Design review of the part built by this model. Coordinates are the model's own, in mm. A direction names the side the tool comes from. Round coordinates to 2 decimals unless told otherwise and drop trailing zeros. Write each loop counter-clockwise with the first axis right and the second up, starting at its lowest first coordinate (ties: lowest second). Pieces come first, ordered by that corner, then holes. Notation, with made-up numbers: M 28.25,-5.75 L 81.25,-5.75 A13 cw 81.25,-1.75 Z; hole C -6.5,7 d6. An arc over 180 degrees is marked long. One line per question, with ' | ' between items. Start each with the question number.
Item 1: For L1, parallel to Y at x = 42, z = 2.35; L2, parallel to Y at x = 41.25, z = 0.75; L3, parallel to X at y = 115, z = 1.55, list the stretches that pass through material, from the lowest coordinate up.
Item 2: Draft analysis for pull direction X (two halves, no side actions). For faces 3 (the face through (-1, 5, 0)), 4 (the face through (-37.591, 123.862, 1.479)), state which applies: released by +X, released by -X, zero draft, split by the parting line, or undercut.
Item 3: Add section A-A, the plane x = -6. State the section outline as (y, z) points, and give its area (3 significant figures).
Item 4: Machinability: for faces 1 (the face through (37.591, 49.138, 1.479)), 2 (the face through (-1, 5, 3)), which of the approach directions +Z, -Z, +X, -X, +Y, -Y give a long, thin tool a straight path to every point of the face, cutting with its end or side? Answer none if there is none.
Item 5: Add section B-B, the plane z = 1.05. Give the number of separate pieces and of enclosed holes in the cut face, and give its area (3 significant figures).
Autodesk Inventor part; units mm, degrees
ref_plane "YZ Plane" through (0, 0, 0) normal (1, 0, 0) x (0, 1, 0)
ref_plane "XZ Plane" through (0, 0, 0) normal (0, 1, 0) x (-1, 0, 0)
ref_plane "XY Plane" through (0, 0, 0) normal (0, 0, 1) x (1, 0, 0)
sketch "スケッチ1" plane through (0, 0, 0) normal (0, 0, 1) x (1, 0, 0)
  line L0 (-55, -225) -> (55, -225)
  line L1 (55, -225) -> (55, 225)
  line L2 (55, 225) -> (-55, 225)
  line L3 (-55, 225) -> (-55, -225)
  line L4 (-55, -225) -> (55, 225) construction
  line L5 (55, -225) -> (-55, 225) construction
  line L6 (-55, 195) -> (-50, 195) construction
  line L7 (-50, 195) -> (-25, 220) construction
  line L8 (-25, 220) -> (-25, 225) construction
  line L9 (-46, 40.5) -> (46, 40.5) construction
  line L10 (46, 40.5) -> (46, 132.5) construction
  line L11 (46, 132.5) -> (-46, 132.5) construction
  line L12 (-46, 132.5) -> (-46, 40.5) construction
  line L13 (-46, 40.5) -> (46, 132.5) construction
  line L14 (46, 40.5) -> (-46, 132.5) construction
  line L15 (-46, 1.5) -> (46, 1.5) construction
  line L16 (46, 1.5) -> (46, 37.5) construction
  line L17 (46, 37.5) -> (-46, 37.5) construction
  line L18 (-46, 37.5) -> (-46, 1.5) construction
  line L19 (-46, 1.5) -> (46, 37.5) construction
  line L20 (46, 1.5) -> (-46, 37.5) construction
  line L21 (0, 0) -> (0, 86.5) construction
  circle A0 centre (0, 86.5) radius 53 construction
  line L22 (-44.7, 41.8) -> (44.7, 41.8) construction
  line L23 (44.7, 41.8) -> (44.7, 131.2) construction
  line L24 (44.7, 131.2) -> (-44.7, 131.2) construction
  line L25 (-44.7, 131.2) -> (-44.7, 41.8) construction
  line L26 (-44.7, 41.8) -> (44.7, 131.2) construction
  line L27 (44.7, 41.8) -> (-44.7, 131.2) construction
  arc A1 (-28.4765, 131.2) -> (-44.7, 114.9765) centre (0, 86.5) ccw
  arc A2 (-44.7, 58.0235) -> (-28.4765, 41.8) centre (0, 86.5) ccw
  arc A3 (28.4765, 41.8) -> (44.7, 58.0235) centre (0, 86.5) ccw
  arc A4 (44.7, 114.9765) -> (28.4765, 131.2) centre (0, 86.5) ccw
  line L28 (-28.4765, 131.2) -> (28.4765, 131.2)
  line L29 (-44.7, 114.9765) -> (-44.7, 58.0235)
  line L30 (-28.4765, 41.8) -> (28.4765, 41.8)
  line L31 (44.7, 58.0235) -> (44.7, 114.9765)
  line L32 (-41.25, 45.25) -> (41.25, 45.25) construction
  line L33 (41.25, 45.25) -> (41.25, 127.75) construction
  line L34 (41.25, 127.75) -> (-41.25, 127.75) construction
  line L35 (-41.25, 127.75) -> (-41.25, 45.25) construction
  line L36 (-41.25, 45.25) -> (41.25, 127.75) construction
  line L37 (41.25, 45.25) -> (-41.25, 127.75) construction
  circle A5 centre (-41.25, 127.75) radius 2.25
  circle A6 centre (-41.25, 45.25) radius 2.25
  circle A7 centre (41.25, 45.25) radius 2.25
  circle A8 centre (41.25, 127.75) radius 2.25
  circle A9 centre (-45, 215) radius 2.25
  circle A10 centre (45, 215) radius 2.25
  circle A11 centre (45, -215) radius 2.25
  circle A12 centre (-45, -215) radius 2.25
  circle A13 centre (-45, 0) radius 2.25 construction
  circle A14 centre (45, 0) radius 2.25 construction
  line L38 (-55, 0) -> (55, 0) construction
  circle A15 centre (-41.25, -49.75) radius 2.25
  arc A16 (-44.7, -36.9765) -> (-28.4765, -53.2) centre (0, -8.5) ccw
  line L39 (-28.4765, -53.2) -> (28.4765, -53.2)
  arc A17 (28.4765, -53.2) -> (44.7, -36.9765) centre (0, -8.5) ccw
  circle A18 centre (41.25, -49.75) radius 2.25
  line L40 (44.7, -36.9765) -> (44.7, 19.9765)
  circle A19 centre (41.25, 32.75) radius 2.25
  arc A20 (44.7, 19.9765) -> (28.4765, 36.2) centre (0, -8.5) ccw
  line L41 (-28.4765, 36.2) -> (28.4765, 36.2)
  circle A21 centre (-41.25, 32.75) radius 2.25
  arc A22 (-28.4765, 36.2) -> (-44.7, 19.9765) centre (0, -8.5) ccw
  line L42 (-44.7, 19.9765) -> (-44.7, -36.9765)
  circle A23 centre (-41.25, -144.75) radius 2.25
  arc A24 (-44.7, -131.9765) -> (-28.4765, -148.2) centre (0, -103.5) ccw
  line L43 (-28.4765, -148.2) -> (28.4765, -148.2)
  arc A25 (28.4765, -148.2) -> (44.7, -131.9765) centre (0, -103.5) ccw
  circle A26 centre (41.25, -144.75) radius 2.25
  line L44 (44.7, -131.9765) -> (44.7, -75.0235)
  circle A27 centre (41.25, -62.25) radius 2.25
  arc A28 (44.7, -75.0235) -> (28.4765, -58.8) centre (0, -103.5) ccw
  line L45 (-28.4765, -58.8) -> (28.4765, -58.8)
  circle A29 centre (-41.25, -62.25) radius 2.25
  arc A30 (-28.4765, -58.8) -> (-44.7, -75.0235) centre (0, -103.5) ccw
  line L46 (-44.7, -75.0235) -> (-44.7, -131.9765)
  point P0 (0, 19.5)
  point P1 (0, 19.5)
  dimension "d12" = 106
  dimension "d0" = 110
  dimension "d1" = 450
  dimension "d2" = 135
  dimension "d3" = 30
  dimension "d4" = 30
  dimension "d5" = 5
  dimension "d6" = 92
  dimension "d7" = 92
  dimension "d8" = 92
  dimension "d9" = 36
  dimension "d10" = 3
  dimension "d11" = 1.5
  dimension "d13" = 89.4
  dimension "d14" = 89.4
  dimension "d15" = 82.5
  dimension "d16" = 82.5
  dimension "d17" = 4.5
  dimension "d25" = 4.5
  dimension "d26" = 10
  dimension "d27" = 10
  dimension "d28" = 10
  dimension "d29" = 10
  dimension "d30" = 10
  dimension "d31" = 10
  dimension "d32" = 10
  dimension "d33" = 10
  dimension "d34" = 10
  dimension "d35" = 10
  dimension "d45" = 95
extrude "押し出し1" add sketch "スケッチ1" along normal blind 3 contours L3 L2 L1 L0 | A15 | L42 A22 L41 A20 L40 A17 L39 A16 | A18 | A19 | A21 | A23 | L46 A30 L45 A28 L44 A25 L43 A24 | A26 | A27 | A29
sketch "スケッチ2" plane through (0, 0, 3) normal (0, 0, 1) x (1, 0, 0)
  circle A0 centre (-45, 215) radius 2.25 construction
  circle A1 centre (45, -215) radius 2.25 construction
  circle A2 centre (-45, -215) radius 2.25 construction
  circle A3 centre (-43, 213) radius 2.75 construction
  line L0 (55, 225) -> (-55, 225)
  line L1 (-55, 225) -> (-55, -225)
  line L2 (-43.7153, 216.8472) -> (-41.4298, 215.2577)
  line L3 (-45.2577, 211.4298) -> (-46.8472, 213.7153)
  circle A4 centre (-45, 215) radius 2.25 construction
  arc A5 (-43.7153, 216.8472) -> (-46.8472, 213.7153) centre (-45, 215) ccw
  arc A6 (-45.2577, 211.4298) -> (-41.4298, 215.2577) centre (-43, 213) ccw
  line L4 (55, 225) -> (-55, 225) construction
  line L5 (0, 225) -> (0, -225) construction
  line L6 (-55, -225) -> (55, -225) construction
  line L7 (-55, 0) -> (55, 0) construction
  line L8 (55, -225) -> (55, 225) construction
  circle A7 centre (45, 215) radius 2.25 construction
  circle A8 centre (43, 213) radius 2.75 construction
  line L9 (43.7153, 216.8472) -> (41.4298, 215.2577)
  line L10 (45.2577, 211.4298) -> (46.8472, 213.7153)
  circle A9 centre (45, 215) radius 2.25 construction
  arc A10 (46.8472, 213.7153) -> (43.7153, 216.8472) centre (45, 215) ccw
  arc A11 (41.4298, 215.2577) -> (45.2577, 211.4298) centre (43, 213) ccw
  circle A12 centre (-45, -215) radius 2.25 construction
  circle A13 centre (-43, -213) radius 2.75 construction
  line L11 (-43.7153, -216.8472) -> (-41.4298, -215.2577)
  line L12 (-45.2577, -211.4298) -> (-46.8472, -213.7153)
  circle A14 centre (-45, -215) radius 2.25 construction
  arc A15 (-46.8472, -213.7153) -> (-43.7153, -216.8472) centre (-45, -215) ccw
  arc A16 (-41.4298, -215.2577) -> (-45.2577, -211.4298) centre (-43, -213) ccw
  circle A17 centre (45, -215) radius 2.25 construction
  line L13 (45.2577, -211.4298) -> (46.8472, -213.7153)
  arc A18 (45.2577, -211.4298) -> (41.4298, -215.2577) centre (43, -213) ccw
  circle A19 centre (43, -213) radius 2.75 construction
  line L14 (43.7153, -216.8472) -> (41.4298, -215.2577)
  circle A20 centre (45, -215) radius 2.25 construction
  arc A21 (43.7153, -216.8472) -> (46.8472, -213.7153) centre (45, -215) ccw
  point P0 (0, 0)
  dimension "d38" = 5.5
  dimension "d39" = 12
  dimension "d40" = 12
extrude "押し出し2" cut sketch "スケッチ2" against normal through all
sketch "スケッチ3" plane through (0, 0, 3) normal (0, 0, 1) x (1, 0, 0)
  line L0 (-55, -225) -> (55, -225) construction
  line L1 (-55, -221.5) -> (55, -221.5)
  line L2 (55, -221.5) -> (55, -225)
  line L3 (55, -225) -> (-55, -225)
  line L4 (-55, -225) -> (-55, -221.5)
  line L5 (-55, -221.5) -> (55, -225) construction
  line L6 (55, -221.5) -> (-55, -225) construction
  line L7 (0, -223.25) -> (0, -225) construction
  point P0 (0, 0)
  dimension "d50" = 3.5
  dimension "d51" = 110
extrude "押し出し3" cut sketch "スケッチ3" against normal through all
sketch "スケッチ4" plane through (0, 0, 3) normal (0, 0, 1) x (1, 0, 0)
  line L0 (-55, -221.5) -> (55, -221.5) construction
  line L1 (55, -221.5) -> (55, 225) construction
  line L2 (55, 225) -> (-55, 225) construction
  line L3 (-55, 225) -> (-55, -221.5) construction
  circle A0 centre (-41.25, 127.75) radius 2.25 construction
  circle A1 centre (-41.25, 45.25) radius 2.25 construction
  circle A2 centre (41.25, 45.25) radius 2.25 construction
  circle A3 centre (41.25, 127.75) radius 2.25 construction
  line L4 (43.7153, -216.8472) -> (41.4298, -215.2577) construction
  arc A4 (45.2577, -211.4298) -> (41.4298, -215.2577) centre (43, -213) ccw construction
  line L5 (45.2577, -211.4298) -> (46.8472, -213.7153) construction
  arc A5 (43.7153, -216.8472) -> (46.8472, -213.7153) centre (45, -215) ccw construction
  line L6 (-28.4765, 131.2) -> (28.4765, 131.2) construction
  arc A6 (44.7, 114.9765) -> (28.4765, 131.2) centre (0, 86.5) ccw construction
  line L7 (44.7, 114.9765) -> (44.7, 58.0235) construction
  arc A7 (28.4765, 41.8) -> (44.7, 58.0235) centre (0, 86.5) ccw construction
  line L8 (28.4765, 41.8) -> (-28.4765, 41.8) construction
  arc A8 (-44.7, 58.0235) -> (-28.4765, 41.8) centre (0, 86.5) ccw construction
  line L9 (-44.7, 58.0235) -> (-44.7, 114.9765) construction
  arc A9 (-28.4765, 131.2) -> (-44.7, 114.9765) centre (0, 86.5) ccw construction
  line L10 (41.4298, 215.2577) -> (43.7153, 216.8472) construction
  arc A10 (46.8472, 213.7153) -> (43.7153, 216.8472) centre (45, 215) ccw construction
  line L11 (46.8472, 213.7153) -> (45.2577, 211.4298) construction
  arc A11 (41.4298, 215.2577) -> (45.2577, 211.4298) centre (43, 213) ccw construction
  line L12 (-45.2577, 211.4298) -> (-46.8472, 213.7153) construction
  arc A12 (-43.7153, 216.8472) -> (-46.8472, 213.7153) centre (-45, 215) ccw construction
  line L13 (-43.7153, 216.8472) -> (-41.4298, 215.2577) construction
  arc A13 (-45.2577, 211.4298) -> (-41.4298, 215.2577) centre (-43, 213) ccw construction
  line L14 (-41.4298, -215.2577) -> (-43.7153, -216.8472) construction
  arc A14 (-46.8472, -213.7153) -> (-43.7153, -216.8472) centre (-45, -215) ccw construction
  line L15 (-46.8472, -213.7153) -> (-45.2577, -211.4298) construction
  arc A15 (-41.4298, -215.2577) -> (-45.2577, -211.4298) centre (-43, -213) ccw construction
  line L16 (-54.75, -221.25) -> (54.75, -221.25)
  line L17 (54.75, -221.25) -> (54.75, 224.75)
  line L18 (54.75, 224.75) -> (-54.75, 224.75)
  line L19 (-54.75, 224.75) -> (-54.75, -221.25)
  point P0 (0, 0)
  dimension "d54" = 0.25
extrude "押し出し4" [suppressed]
equation "\"d4\" = d3"
equation "\"d11\" = 0.5 * d10"
equation "\"d27\" = d26"
equation "\"d28\" = d26"
equation "\"d29\" = d26"
equation "\"d30\" = d26"
equation "\"d31\" = d26"
equation "\"d32\" = d26"
equation "\"d33\" = d26"
equation "\"d34\" = d26"
equation "\"d35\" = d26"
equation "\"d45\" = d7 + d10"
properties part number "bottom_panel" material "アルミニウム 6061"
Computed values:
1) L1: y = -221.5 to -215.65, -210.44 to 43.13, 47.37 to 54.17, 118.83 to 125.63, 129.87 to 210.44, 215.65 to 225 | L2: y = -221.5 to -215.12, -210.88 to 43, 47.5 to 53.22, 119.78 to 125.5, 130 to 210.88, 215.12 to 225 | L3: x = -55 to -44.69, 44.69 to 55
2) face 3: zero draft | face 4: undercut
3) outline: M -221.5,0 L 41.8,0 L 41.8,3 L -221.5,3 Z; M 131.2,0 L 225,0 L 225,3 L 131.2,3 Z | area: 1,070 mm^2
4) face 1: +Z, -Z | face 2: +Z, +X, -X, +Y, -Y
5) separate pieces: 1 | enclosed holes: 9 | area: 41,400 mm^2
